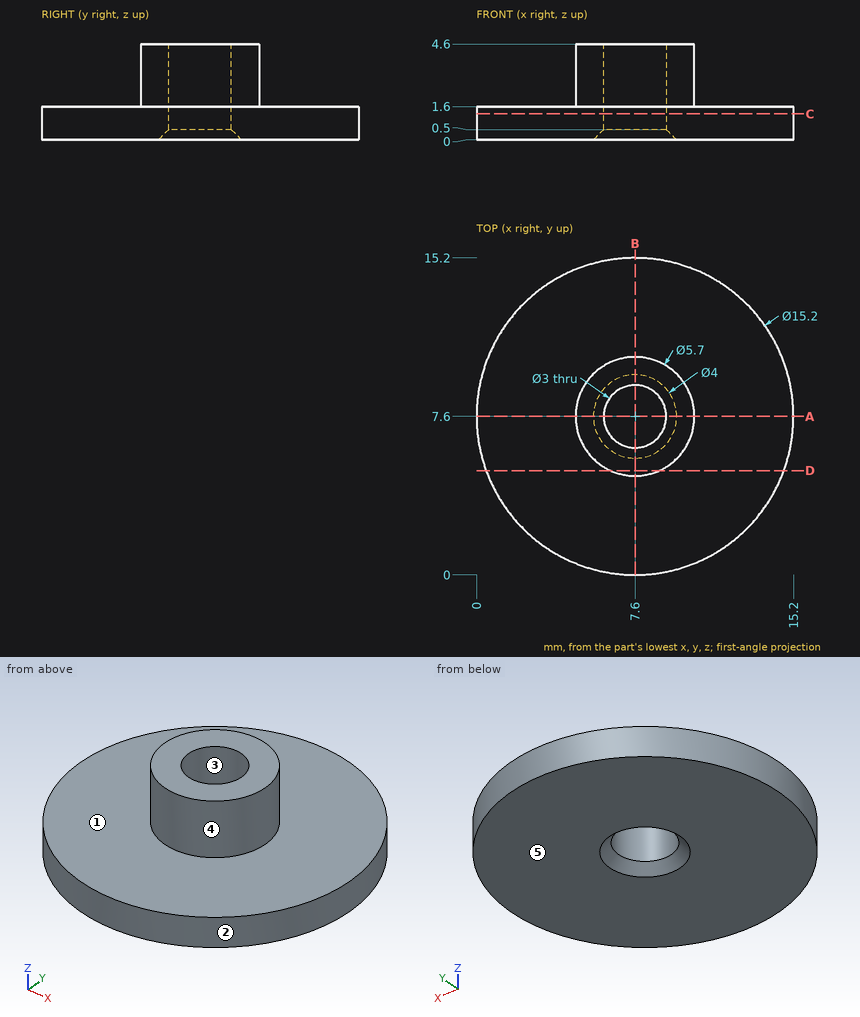
Study the drawing (mm; zero at the part's minimum x, y, z) and answer. A direction names the side the tool comes from. Coordinates: 2 decimals unless noted, no trailing zeros. Write each loop counter-clockwise with the first axis right and the second up, starting at its lowest first coordinate (ties: lowest second). Pieces come first, ordered by that corner, then holes.
Q1. Determine the mould class of the marked faces 3, 4 and 5 for opening direction X: released by +X, released by -X, zero draft, split by the parting line, or undercut.
Q2. A cutting plane is placed at D-D, the plane y = 5. Give the vertices of the cut face in (x, z).
Q3. Each of these flat-tipped pins is pushed along its axis until it touches: pin 1 Ø6 at (x, y) = (5, 13) entering from +Z; pin 2 Ø2.5 at (x, y) = (7.6, 7.6) entering from -Z; pin 3 Ø1.5 at (x, z) = (8.5, 2.5) entering from +Y. Where does it stop, or does it pass through?
Q4. Which of the six approach directions +Z, -Z, +X, -X, +Y, -Y give full straight-line access (tool end or side, diameter ignored) to the marked faces 1 and 2?
Q5. Find the intervals of material crossed by line 1 (Y direction, x = 7.6, z = 2.4); line 2 (Y direction, x = 7.6, z = 1.4); line 3 (Z direction, x = 5.25, y = 10.5), in increasing order.
Q6. A cutting plane is placed at C-C, the plane z = 1.25. Give the vertices of the cut face in (x, y).
Q7. A cutting plane is placed at A-A, the plane y = 7.6. Give the vertices of the cut face in (x, z), then the cut area to 3 significant figures.
Findings below:
1. face 3: undercut
1. face 4: split by the parting line
1. face 5: zero draft
2. outline: (0.46, 0) - (14.74, 0) - (14.74, 1.6) - (8.77, 1.6) - (8.77, 4.6) - (6.43, 4.6) - (6.43, 1.6) - (0.46, 1.6) - close
3. pin 1: stops at z = 1.6
3. pin 2: passes through
3. pin 3: stops at y = 10.45
4. face 1: +Z
4. face 2: +Z, -Z
5. line 1: y = 4.75 to 6.1, 9.1 to 10.45
5. line 2: y = 0 to 6.1, 9.1 to 15.2
5. line 3: z = 0 to 1.6
6. outline: circle Ø15.2 at (7.6, 7.6); hole circle Ø3 at (7.6, 7.6)
7. outline: (0, 0) - (5.6, 0) - (6.1, 0.5) - (6.1, 4.6) - (4.75, 4.6) - (4.75, 1.6) - (0, 1.6) - close; (9.1, 0.5) - (9.6, 0) - (15.2, 0) - (15.2, 1.6) - (10.45, 1.6) - (10.45, 4.6) - (9.1, 4.6) - close
7. area: 27.4 mm2
